The listing builds one solid part. Answer for the finished solid, in the listing's coordinates (mm). A direction names the side the tool comes from. Round coordinates to 2 decimals unless told otherwise and drop trailing zeros. Loops run counter-clockwise (first coordinate to the right, second up) from the corner with the lowest first, then second, coordinate; pieces in that order, holes last. Notation, with made-up numbers: (82, 46.25) - (126, 46.25) arc R7 cw to (126, 54.25) - close; hole circle Ø4 at (77, 84.25). An arc over 180 degrees is marked (long way). One line per question, with ' | ' between items. Start each with the question number.
from build123d import *

# Parameters (mm, degrees)
SKICA1_W                 = 12.5
SKICA1_H                 = 24.3
P_IDAT_VYSUNUT_M1_DEPTH  = 4.52
ODEBRAT_VYSUNUT_M1_DEPTH = 4.52
ODEBRAT_VYSUNUT_M2_DEPTH = 4.52
ZAOBLIT1_R               = 1
ZAOBLIT2_R               = 3
P_IDAT_VYSUNUT_M2_DEPTH  = 6.174
ZAOBLIT4_R               = 1
ODEBRAT_VYSUNUT_M3_DEPTH = 2


with BuildPart() as part:
    # Skica1 → Přidat vysunutím1 (new body)
    with BuildSketch(Plane.XY):
        Rectangle(SKICA1_W, SKICA1_H)
    extrude(amount=P_IDAT_VYSUNUT_M1_DEPTH)

    # Skica2 → Odebrat vysunutím1 (cut)
    with BuildSketch(Plane(origin=(0, 0, 0), x_dir=(-1, 0, 0), z_dir=(0, 0, -1))):
        with BuildLine():
            Line((-6.25, 12.15), (-6.25, 8.95))
            ThreePointArc((-6.25, 8.95), (-3.510786949, 11.303490134), (0, 12.15))
            Line((0, 12.15), (-6.25, 12.15))
        make_face()
        with BuildLine():
            Line((6.25, 12.15), (0, 12.15))
            ThreePointArc((0, 12.15), (3.510786949, 11.303490134), (6.25, 8.95))
            Line((6.25, 8.95), (6.25, 12.15))
        make_face()
    extrude(amount=-ODEBRAT_VYSUNUT_M1_DEPTH, mode=Mode.SUBTRACT)

    # Skica3 → Odebrat vysunutím2 (cut)
    with BuildSketch(Plane(origin=(0, 0, 0), x_dir=(-1, 0, 0), z_dir=(0, 0, -1))):
        with BuildLine():
            Line((-6.25, -10.10590929), (-6.25, -12.15))
            Line((-6.25, -12.15), (-5.130314287, -12.15))
            ThreePointArc((-5.130314287, -12.15), (-5.519629341, -11.034545119), (-6.25, -10.10590929))
        make_face()
        with BuildLine():
            Line((6.25, -12.15), (5.130314287, -12.15))
            ThreePointArc((5.130314287, -12.15), (5.519629341, -11.034545119), (6.25, -10.10590929))
            Line((6.25, -10.10590929), (6.25, -12.15))
        make_face()
    extrude(amount=-ODEBRAT_VYSUNUT_M2_DEPTH, mode=Mode.SUBTRACT)

    # Zaoblit1
    zaoblit1_edges = [part.edges().sort_by_distance(p)[0] for p in [
        (6.25, -10.10590929, 2.26),
        (5.130314287, -12.15, 2.26),
        (-5.130314287, -12.15, 2.26),
        (-6.25, -10.10590929, 2.26),
    ]]
    fillet(zaoblit1_edges, radius=ZAOBLIT1_R)

    # Zaoblit2
    zaoblit2_edges = [part.edges().sort_by_distance(p)[0] for p in [
        (6.25, 8.95, 2.26),
        (-6.25, 8.95, 2.26),
    ]]
    fillet(zaoblit2_edges, radius=ZAOBLIT2_R)

    # Skica4 → Přidat vysunutím2 (add)
    with BuildSketch(Plane(origin=(0, 0, 0), x_dir=(-1, 0, 0), z_dir=(0, 0, -1))):
        Polygon((0, 11.15), (-5.5, 8.726822139), (-5.5, -8.426822139), (0, -10.85), (5.5, -8.426822139), (5.5, 8.726822139), align=None)
    extrude(amount=P_IDAT_VYSUNUT_M2_DEPTH)

    # Zaoblit4
    zaoblit4_edges = [part.edges().sort_by_distance(p)[0] for p in [
        (0, -10.85, -3.087),
        (-5.5, -8.426822139, -3.087),
        (-5.5, 8.726822139, -3.087),
        (0, 11.15, -3.087),
        (5.5, 8.726822139, -3.087),
        (5.5, -8.426822139, -3.087),
    ]]
    fillet(zaoblit4_edges, radius=ZAOBLIT4_R)

    # Skica5 → Odebrat vysunutím3 (cut)
    with BuildSketch(Plane.XY.offset(4.52)):
        with BuildLine():
            Line((6.25, -9.69593403), (6.25, 7.846566614))
            ThreePointArc((6.25, 7.846566614), (6.008509797, 9.025813706), (5.322917532, 10.015209717))
            ThreePointArc((5.322917532, 10.015209717), (0, 12.15), (-5.322917532, 10.015209717))
            ThreePointArc((-5.322917532, 10.015209717), (-6.008509797, 9.025813706), (-6.25, 7.846566614))
            Line((-6.25, 7.846566614), (-6.25, -9.69593403))
            ThreePointArc((-6.25, -9.69593403), (-6.183994107, -10.053222441), (-5.994689983, -10.36334457))
            ThreePointArc((-5.994689983, -10.36334457), (-5.597278437, -10.899802086), (-5.306089821, -11.500578079))
            ThreePointArc((-5.306089821, -11.500578079), (-4.939390465, -11.971759721), (-4.369556313, -12.15))
            Line((-4.369556313, -12.15), (4.369556313, -12.15))
            ThreePointArc((4.369556313, -12.15), (4.939390465, -11.971759721), (5.306089821, -11.500578079))
            ThreePointArc((5.306089821, -11.500578079), (5.597278437, -10.899802086), (5.994689983, -10.36334457))
            ThreePointArc((5.994689983, -10.36334457), (6.183994107, -10.053222441), (6.25, -9.69593403))
        make_face()
    extrude(amount=-ODEBRAT_VYSUNUT_M3_DEPTH, mode=Mode.SUBTRACT)


solid = part.part
(1) Find section B-B on x = -0.75. Write down the section's boundary in (y, z).
(2) Each of these flat-tipped pins is pushed along its axis until it touches: P1, Ø1.5, axis at x = 1.5, z = -1.5, coming from the +Y side; P2, Ø1.9, axis at y = 3.5, z = -3.5, coming from the -X side; P3, Ø1.5, axis at y = -1.5, z = -4.5, coming from the +X side. Where does it stop, or does it pass through?
(3) Consider L1, parallel to X at y = -1.75, z = -0.75; L2, parallel to Z at x = 5.5, y = -8.25; L3, parallel to X at y = -9.25, z = -0.5. Determine where each line is inside the solid, lowest interval first.
(4) Find section C-C on y = -3.5. Write down the section's boundary in (x, z), plus the area to 3 significant figures.
(5) A tool of negligible diameter and unlimited length cuts with its end or side. For faces 1 (the flat face through (5.5, 0, -3)), 2 (the cylindrical face through (5.342, 8.614, -3.13)), 3 (the cylindrical face through (-0.006, 11.057, -3.13)), 4 (the cylindrical face through (-0.006, -10.757, -3.13)), from which of +Z, -Z, +X, -X, +Y, -Y can it reach the whole face along a straight path? Write none if from no direction.
(6) Find section A-A on z = -2.25. Write down the section's boundary in (x, y).
Answer below:
1) outline: (-12.15, 0) - (-10.52, 0) - (-10.52, -6.17) - (10.82, -6.17) - (10.82, 0) - (12.11, 0) - (12.11, 2.52) - (-12.15, 2.52) - close
2) P1: y = 10.82 | P2: x = -5.5 | P3: x = 5.5
3) L1: -5.5 to 5.5 | L2: 0 to 2.52 | L3: -3.63 to 3.63
4) outline: (-6.25, 0) - (-5.5, 0) - (-5.5, -6.17) - (5.5, -6.17) - (5.5, 0) - (6.25, 0) - (6.25, 2.52) - (-6.25, 2.52) - close | area: 99.4 mm2
5) face 1: -Z, +X, +Y, -Y | face 2: -Z, +X, +Y | face 3: -Z, +Y | face 4: -Z, -Y
6) outline: (-5.5, -7.77) arc R1 ccw to (-4.9, -8.69) - (-0.4, -10.67) arc R1 ccw to (0.4, -10.67) - (4.9, -8.69) arc R1 ccw to (5.5, -7.77) - (5.5, 8.07) arc R1 ccw to (4.9, 8.99) - (0.4, 10.97) arc R1 ccw to (-0.4, 10.97) - (-4.9, 8.99) arc R1 ccw to (-5.5, 8.07) - close
